Drawing for the job (mm, zero at the part's lowest x, y, z). Coordinates: 2 decimals unless noted, no trailing zeros. Order: outer loops, then holes, each group sorted by start corner. A loop starts at its lowest first (then second) coordinate and runs counter-clockwise, first axis right, second up. Notation, with made-up numbers: (68, 1) - (73, 1) arc R19 ccw to (73, 22) - close; hole circle Ø8 at (85.25, 37.25). An arc over 180 degrees is marked (long way). Put each result on its own line as item: value. Start each with the question number.
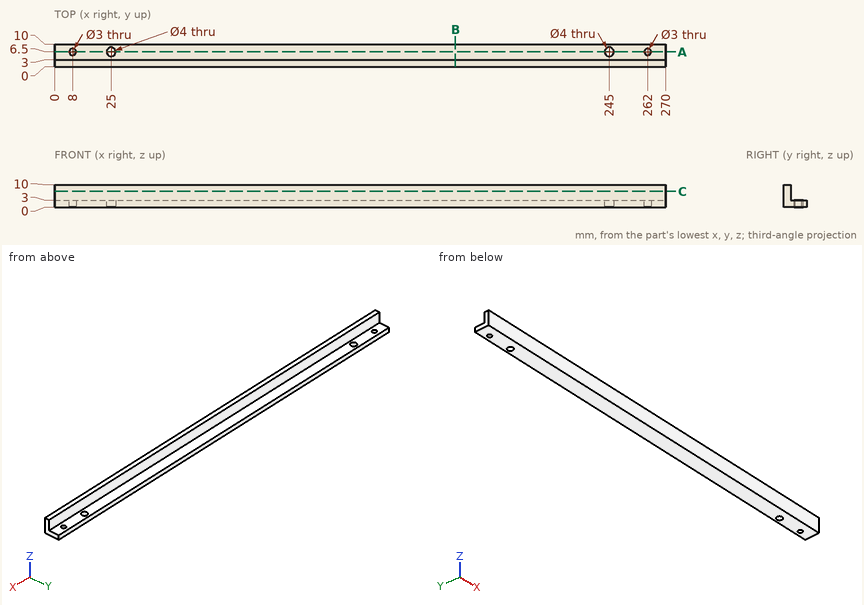
Item 1: Flat gauge pins, fed straight in: pin 1 Ø1.5 at (x, z) = (145, 8) entering from +Y; pin 2 Ø3 at (x, y) = (245, 6.5) entering from -Z. Where does each tip first touch, or does it go through?
Item 2: Wall check: line 1 along Y through (x, z) = (25, 2.1); line 2 along Y through (x, z) = (262, 1.45); line 3 along X through (y, z) = (7.5, 1.5). Give the ranges that are in metal, low to high.
Item 3: Slice it at C-C, the plane z = 7. Give the cut face in (x, y).
Item 4: Slice it at A-A, the plane y = 6.5. Give the cut face in (x, z), plus the area to 3 significant figures.
Item 5: Slice it at B-B, the plane x = 177. Give the cut face in (y, z), plus the area to 3 significant figures.
Here are the results:
1. pin 1: stops at y = 3
1. pin 2: passes through
2. line 1: y = 0 to 4.5, 8.5 to 10
2. line 2: y = 0 to 5, 8 to 10
2. line 3: x = 0 to 6.88, 9.12 to 23.27, 26.73 to 243.27, 246.73 to 260.88, 263.12 to 270
3. outline: (0, 0) - (270, 0) - (270, 3) - (0, 3) - close
4. outline: (0, 0) - (6.5, 0) - (6.5, 3) - (0, 3) - close; (9.5, 0) - (23, 0) - (23, 3) - (9.5, 3) - close; (27, 0) - (243, 0) - (243, 3) - (27, 3) - close; (247, 0) - (260.5, 0) - (260.5, 3) - (247, 3) - close; (263.5, 0) - (270, 0) - (270, 3) - (263.5, 3) - close
4. area: 768 mm^2
5. outline: (0, 0) - (10, 0) - (10, 3) - (3, 3) - (3, 10) - (0, 10) - close
5. area: 51.0 mm^2
